```python
from build123d import *

# Parameters (mm, degrees)
SKETCH1_W           = 12
SKETCH1_H           = 11
BOSS_EXTRUDE1_DEPTH = 14
SHELL1_T            = -2
SKETCH2_R           = 0.75
CUT_EXTRUDE1_DEPTH  = 10


with BuildPart() as part:
    # Sketch1 → Boss-Extrude1 (new body)
    with BuildSketch(Plane(origin=(0, 0, 0), x_dir=(1, 0, 0), z_dir=(0, 1, 0))):
        with Locations((6, 5.5)):
            Rectangle(SKETCH1_W, SKETCH1_H)
    extrude(amount=BOSS_EXTRUDE1_DEPTH)

    # Shell1
    shell1_openings = [part.faces().sort_by_distance(p)[0] for p in [
        (6, 14, -5.5),
    ]]
    offset(amount=SHELL1_T, openings=shell1_openings, kind=Kind.INTERSECTION)

    # Sketch2 → Cut-Extrude1 (cut)
    with BuildSketch(Plane.XZ):
        with Locations((3.452899673, -7.28987771)):
            Circle(SKETCH2_R)
        with Locations((5.992899673, -7.28987771)):
            Circle(SKETCH2_R)
        with Locations((8.532899673, -7.28987771)):
            Circle(SKETCH2_R)
    extrude(amount=-CUT_EXTRUDE1_DEPTH, mode=Mode.SUBTRACT)


solid = part.part
```
Can you work these out from the model? Positions are in its coordinate system, mm. A direction names the side the tool comes from. Round coordinates to 2 decimals unless told otherwise and drop trailing zeros. Loops run counter-clockwise (first coordinate to the right, second up) from the corner with the lowest first, then second, coordinate; pieces in that order, holes last.
Item 1: Suppose I cut it at A-A, the plane x = 4. Write out the boundary of the cut face in (y, z).
Item 2: Suppose I cut it at B-B, the plane y = 6. Write out the boundary of the cut face in (x, z), then the cut area to 3 significant figures.
Item 3: Suppose I cut it at D-D, the plane z = -7.75. Write out the boundary of the cut face in (x, y), then the cut area to 3 significant figures.
Item 4: Please list where these lines run through material, in increasing order: L1, parallel to Z at x = 6, y = 7.5; L2, parallel to X at y = 4, z = -7.75; L3, parallel to Z at x = 9, y = 1.25.
Item 5: Suppose I cut it at C-C, the plane z = -2.75. Write out the boundary of the cut face in (x, y), then the cut area to 3 significant figures.
Item 6: If we mould it in two halves opening along X, with no side actions, what happens to faces 1 (the flat face through (0, 7, -5)), 2 (the cylindrical face through (3.86, 0.99, -6.66)), 3 (the flat face through (6, 7, 0))? For each: +X half, -X half, draft (parallel to the pull), parting line (faces both ways), or undercut.
Item 7: Which directions (+Z, -Z, +X, -X, +Y, -Y) give clear straight access to the entire face, cutting with the end or side of a thin tool? Please do faces 4 (the cylindrical face through (5.895, 0.986, -6.546)), 5 (the flat face through (6, 8, -2)).
Reported:
1. outline: (0, -11) - (14, -11) - (14, -9) - (2, -9) - (2, -7.8) - (0, -7.8) - close; (0, -6.78) - (2, -6.78) - (2, -2) - (14, -2) - (14, 0) - (0, 0) - close
2. outline: (0, -11) - (12, -11) - (12, 0) - (0, 0) - close; hole (2, -9) - (10, -9) - (10, -2) - (2, -2) - close
2. area: 76.0 mm2
3. outline: (0, 0) - (2.86, 0) - (2.86, 2) - (2, 2) - (2, 14) - (0, 14) - close; (4.05, 0) - (5.4, 0) - (5.4, 2) - (4.05, 2) - close; (6.59, 0) - (7.94, 0) - (7.94, 2) - (6.59, 2) - close; (9.13, 0) - (12, 0) - (12, 14) - (10, 14) - (10, 2) - (9.13, 2) - close
3. area: 64.9 mm2
4. L1: z = -11 to -9, -2 to 0
4. L2: x = 0 to 2, 10 to 12
4. L3: z = -11 to -7.88, -6.7 to 0
5. outline: (0, 0) - (12, 0) - (12, 14) - (10, 14) - (10, 2) - (2, 2) - (2, 14) - (0, 14) - close
5. area: 72.0 mm2
6. face 1: -X half
6. face 2: undercut
6. face 3: draft
7. face 4: +Y, -Y
7. face 5: +Y
